from build123d import *

# Parameters (mm, degrees)
F0_W     = 20
F0_H     = 20
F0_W_2   = 40
F0_H_2   = 30
F1_DEPTH = 60
F3_W     = 50
F3_H     = 20
F4_DEPTH = 10


with BuildPart() as f1:
    # F0 (on Front) → F1 (new body)
    with BuildSketch(Plane.XZ):
        Polygon((49.277523, 25.879864), (-50.722477, 25.879864), (-50.722477, -4.120136), (-30.722477, -4.120136), (-30.722477, -24.120136), (9.277523, -24.120136), (9.277523, 5.879864), (49.277523, 5.879864), align=None)
        with Locations((-40.722477, -14.120136)):
            Rectangle(F0_W, F0_H)
        with Locations((29.277523, -9.120136)):
            Rectangle(F0_W_2, F0_H_2)
    extrude(amount=-F1_DEPTH)

    # F3 (on face) → F4 (cut)
    with BuildSketch(Plane(origin=(-50.722477, 0, 0), x_dir=(0, -1, 0), z_dir=(-1, 0, 0))):
        with Locations((-29.763764, 15.879864)):
            Rectangle(F3_W, F3_H)
    extrude(amount=-F4_DEPTH, mode=Mode.SUBTRACT)


solid = f1.part
Verification items for the finished model (mm, model axes). A direction names the side the tool comes from. Round coordinates to 2 decimals unless told otherwise and drop trailing zeros. Loops run counter-clockwise (first coordinate to the right, second up) from the corner with the lowest first, then second, coordinate; pieces in that order, holes last. Notation, with made-up numbers: (74.25, 33) - (120.25, 33) arc R27 cw to (120.25, 52) - close; hole circle Ø2 at (50, 59.25). An arc over 180 degrees is marked (long way). Write item = value, one per line.
Q1. Sectioned sample at A-A on z = 18. Record the boundary of the cut face in (x, y), plus the area to 3 significant figures.
Here are the results:
outline = (-50.72, 0) - (49.28, 0) - (49.28, 60) - (-50.72, 60) - (-50.72, 54.76) - (-40.72, 54.76) - (-40.72, 4.76) - (-50.72, 4.76) - close
area = 5,500 mm^2
Q2. Mould release check, pull along Y, two halves, no side actions. Record for faces 3 (the flat face through (-1, 60, 1)), 4 (the flat face through (-46, 30, 5.88)), 5 (the flat face through (-46, 4.764, 16)), 6 (the flat face through (49.278, 30, 1)): +Y half, -Y half, draft (parallel to the pull), parting line (faces both ways), or undercut.
Here are the results:
face_3 = +Y half
face_4 = undercut
face_5 = undercut
face_6 = draft
Q3. Tool access check on faces 1 (the flat face through (-40.722, 30, 16)), 2 (the flat face through (-1, 0, 1)). Record the directions out of +Z, -Z, +X, -X, +Y, -Y that give a thin tool (end or side, any length) a straight path to the whole face; none if there is none.
Here are the results:
face_1 = +Z, -X
face_2 = +Z, -Z, +X, -X, -Y
Q4. Depth check by flat-ended pin: pin 1 (3 mm diameter, centred on x = -44, y = 30, fed in from +Z); pin 2 (10 mm diameter, centred on y = 21, z = 14.5, fed in from -X). Enter the tip coordinate at first touch or a pass-through.
Here are the results:
pin_1 = 5.88
pin_2 = -40.72
Q5. Sectioned sample at B-B on y = 13.5. Record the boundary of the cut face in (x, z).
Here are the results:
outline = (-50.72, -24.12) - (49.28, -24.12) - (49.28, 25.88) - (-40.72, 25.88) - (-40.72, 5.88) - (-50.72, 5.88) - close
Q6. Material ranges on L1, parallel to X at y = 29, z = 12, recorded low to high.
Here are the results:
L1 = -40.72 to 49.28
